Could you check a few things on this drawing? It's one solid part, dimensions in mm from its lowest x, y, z. Give positions to 0.01 mm unless a question says otherwise; leave off trailing zeros. Order: outer loops, then holes, each group sorted by start corner. A loop starts at its lowest first (then second) coordinate and runs counter-clockwise, first axis right, second up. Notation, with made-up numbers: (50.25, 46) - (90.25, 46) arc R16 ccw to (90.25, 58) - close; hole circle Ø3 at (52, 57.25). An arc over 180 degrees is marked (long way). Return JSON: item names as keys, results as strings.
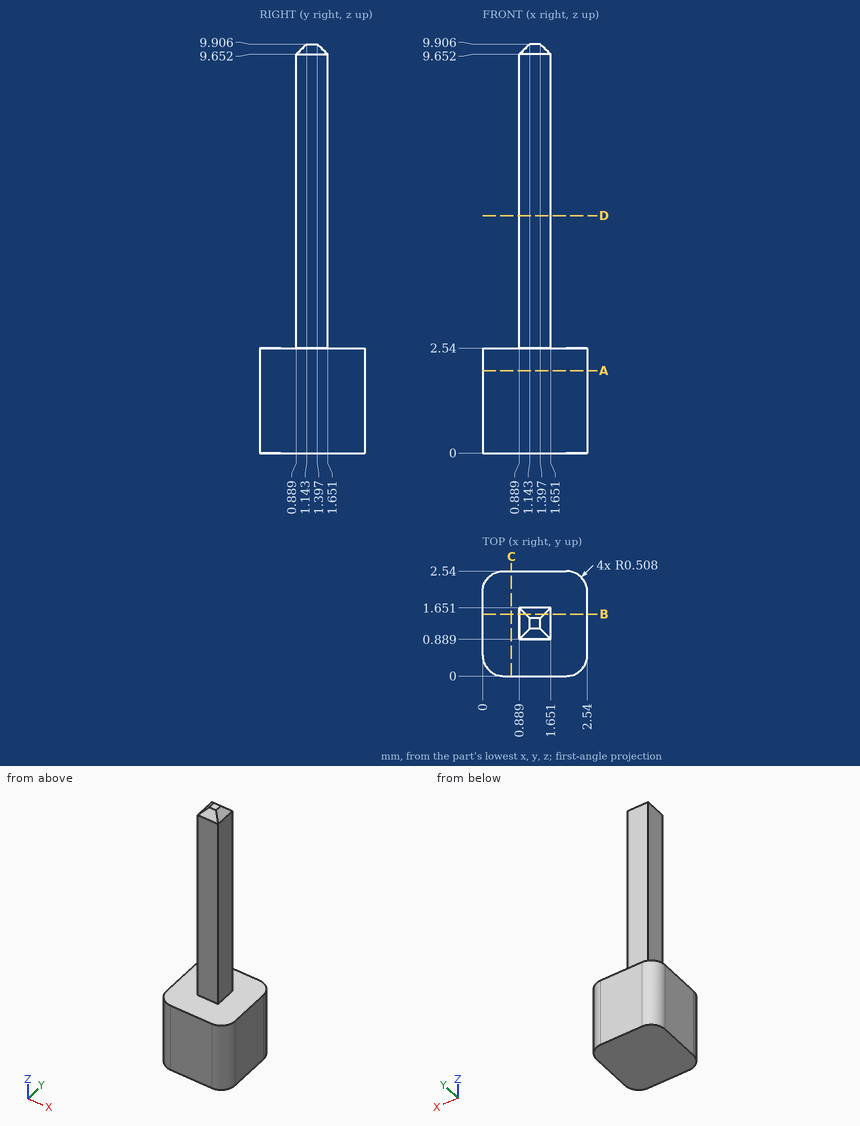
1. For pin 1 Ø1 at (x, z) = (1.5, 6) entering from -Y; pin 2 Ø0.8 at (x, z) = (1.5, 5) entering from +Y; pin 3 Ø1 at (x, z) = (2, 2) entering from -Y; pin 4 Ø1.5 at (y, z) = (1.5, 9) entering from +X, each with a flat end and sliding along its axis, tell me the tip position at first contact or that it passes through.
Checks:
{"pin 1": "y = 0.89", "pin 2": "y = 1.65", "pin 3": "y = 0", "pin 4": "x = 1.65"}
2. Suppose I cut it at A-A (z = 2). List the corners of the cut face in (x, y) for me.
Checks:
{"outline": "(0, 0.51) arc R0.51 ccw to (0.51, 0) - (2.03, 0) arc R0.51 ccw to (2.54, 0.51) - (2.54, 2.03) arc R0.51 ccw to (2.03, 2.54) - (0.51, 2.54) arc R0.51 ccw to (0, 2.03) - close"}
3. If I drill on L1, parallel to Z at x = 2.3, y = 0.35; L2, parallel to X at y = 1.05, z = 3.5, over which ranges is the centre line in solid material (lowest first)? Write a range as [from, to].
Checks:
{"L1": "[0, 2.54]", "L2": "[0.89, 1.65]"}
4. Suppose I cut it at B-B (y = 1.5). List the corners of the cut face in (x, z) for me, plus the area to 3 significant figures.
Checks:
{"outline": "(0, 0) - (2.54, 0) - (2.54, 2.54) - (1.65, 2.54) - (1.65, 9.65) - (1.5, 9.8) - (1.04, 9.8) - (0.89, 9.65) - (0.89, 2.54) - (0, 2.54) - close", "area": "12.0 mm^2"}
5. Suppose I cut it at C-C (x = 0.7). List the corners of the cut face in (y, z) for me.
Checks:
{"outline": "(0, 0) - (2.54, 0) - (2.54, 2.54) - (0, 2.54) - close"}
6. Suppose I cut it at D-D (z = 5.75). List the corners of the cut face in (x, y) for me.
Checks:
{"outline": "(0.89, 0.89) - (1.65, 0.89) - (1.65, 1.65) - (0.89, 1.65) - close"}
